from build123d import *

# Parameters (mm, degrees)
EXTRUDE_1_DEPTH      = 120
EXTRUDE_1_DEPTH_BACK = 120
CHAMFER_1_SIZE       = 4
CHAMFER_1_SIZE_2     = 14.92820323


with BuildPart() as part:
    # Эскиз1 → Вытянуть-Тонкостенный1 (new, two sides: drawn at the far end of the back side and taken through both)
    with BuildSketch(Plane(origin=(0, 0, 0), x_dir=(1, 0, 0), z_dir=(0, 1, 0)).offset(-EXTRUDE_1_DEPTH_BACK)):
        with BuildLine():
            Line((-11, 7.5), (11, 7.5))
            ThreePointArc((11, 7.5), (13.828427125, 6.328427125), (15, 3.5))
            Line((15, 3.5), (15, -3.5))
            ThreePointArc((15, -3.5), (13.828427125, -6.328427125), (11, -7.5))
            Line((11, -7.5), (-11, -7.5))
            ThreePointArc((-11, -7.5), (-13.828427125, -6.328427125), (-15, -3.5))
            Line((-15, -3.5), (-15, 3.5))
            ThreePointArc((-15, 3.5), (-13.828427125, 6.328427125), (-11, 7.5))
        make_face()
        with BuildLine():
            Line((-11, 5.5), (11, 5.5))
            ThreePointArc((11, 5.5), (12.414213562, 4.914213562), (13, 3.5))
            Line((13, 3.5), (13, -3.5))
            ThreePointArc((13, -3.5), (12.414213562, -4.914213562), (11, -5.5))
            Line((11, -5.5), (-11, -5.5))
            ThreePointArc((-11, -5.5), (-12.414213562, -4.914213562), (-13, -3.5))
            Line((-13, -3.5), (-13, 3.5))
            ThreePointArc((-13, 3.5), (-12.414213562, 4.914213562), (-11, 5.5))
        make_face(mode=Mode.SUBTRACT)
    extrude(amount=EXTRUDE_1_DEPTH + EXTRUDE_1_DEPTH_BACK)

    # Фаска1
    # the kernel refuses this chamfer: 14.92820323, 4 mm, written as the material it takes off along each edge
    with BuildSketch(Plane(origin=(-49.764387332, 120, -7.5), x_dir=(0, -0.990500038825954, -0.1375124470212912), z_dir=(1, 0, 0))) as chamfer_1_piece_1:
        Polygon((CHAMFER_1_SIZE * 0.990500038826, -CHAMFER_1_SIZE * 0.137512447021), (-CHAMFER_1_SIZE_2 * 0.137512447024, -CHAMFER_1_SIZE_2 * 0.990500038844), (0, 0), align=None)
    extrude(amount=99.528774665, mode=Mode.SUBTRACT)
    with BuildSketch(Plane(origin=(-49.764387332, -120, -7.5), x_dir=(0, -0.009967146577155871, 0.9999503267608394), z_dir=(1, 0, 0))) as chamfer_1_piece_2:
        Polygon((CHAMFER_1_SIZE_2 * 0.999950326779, -CHAMFER_1_SIZE_2 * 0.00996714657734), (-CHAMFER_1_SIZE * 0.00996714657716, -CHAMFER_1_SIZE * 0.999950326761), (0, 0), align=None)
    extrude(amount=99.528774665, mode=Mode.SUBTRACT)


solid = part.part
Input: part model. Units: mm. Frame: model coordinates. A direction names the side the tool comes from. Round coordinates to 2 decimals unless told otherwise and drop trailing zeros. Order: outer loops, then holes, each group sorted by start corner. A loop starts at its lowest first (then second) coordinate and runs counter-clockwise, first axis right, second up. Notation, with made-up numbers: (32.5, 86.25) - (36.5, 86.25) arc R33 cw to (36.5, 117.25) - close; hole circle Ø10 at (2, 50.5). An arc over 180 degrees is marked (long way). Answer as a JSON object with one key per item and string values. Group by question number.
(1) Cut plane A-A (y = -45). Return loops of the section in (x, z), then the cut area to 3 significant figures.
(2) Cut plane C-C (z = 0.25). Return loops of the section in (x, y), then the cut area to 3 significant figures.
(3) Cut plane B-B (x = 4). Return loops of the section in (y, z), then the cut area to 3 significant figures.
(4) Material intervals for probe 1 along Z at (x, y) = (-9, 104); probe 2 along X at (y, z) = (100.5, 0.5); probe 3 along Y at (x, z) = (11.5, -5.5), sorted ascending. Write a range as from..to.
(5) Draft query along X for faces 1 (the face through (-0.21, -116.25, -6.57)), 2 (the face through (13, -2, 0)), 3 (the face through (15, -2, 0)). Return one class per face: released by +X, released by -X, zero draft, split by the parting line, or undercut.
(6) Reachability of faces 4 (the face through (-13, -2, 0)), 5 (the face through (-13.797, -1.68, 6.359)) from +Z, -Z, +X, -X, +Y, -Y: full face, straight path, thin tool, end or side. Return the list, or none.
Here are the results:
{
 "1": {"outline": "(-15, -3.5) arc R4 ccw to (-11, -7.5) - (11, -7.5) arc R4 ccw to (15, -3.5) - (15, 3.5) arc R4 ccw to (11, 7.5) - (-11, 7.5) arc R4 ccw to (-15, 3.5) - close; hole (-13, -3.5) arc R2 ccw to (-11, -5.5) - (11, -5.5) arc R2 ccw to (13, -3.5) - (13, 3.5) arc R2 ccw to (11, 5.5) - (-11, 5.5) arc R2 ccw to (-13, 3.5) - close", "area": "154 mm^2"},
 "2": {"outline": "(-15, -118.08) - (-13, -118.08) - (-13, 118.08) - (-15, 118.08) - close; (13, -118.08) - (15, -118.08) - (15, 118.08) - (13, 118.08) - close", "area": "945 mm^2"},
 "3": {"outline": "(-120, 7.43) - (-119.48, 5.5) - (119.48, 5.5) - (120, 7.43) - (120, 7.5) - (-120, 7.5) - close; (-116.54, -5.5) - (-116, -7.5) - (116, -7.5) - (116.54, -5.5) - close", "area": "944 mm^2"},
 "4": {"probe 1": "z = -7.5..-5.5, 5.5..7.5", "probe 2": "x = -15..-13, 13..15", "probe 3": "y = -116.54..116.54"},
 "5": {"face 1": "zero draft", "face 2": "undercut", "face 3": "released by +X"},
 "6": {"face 4": "+Y, -Y", "face 5": "+Z, -X, +Y, -Y"}
}
